For this review, take the finished solid that the model builds, in its own axes (mm). A direction names the side the tool comes from. Coordinates: 2 decimals unless noted, no trailing zeros. Write each loop counter-clockwise with the first axis right and the second up, starting at its lowest first coordinate (ties: lowest second). Pieces come first, ordered by that corner, then holes.
```python
from build123d import *

# Parameters (mm, degrees)
SKETCH2_R               = 5
BOSS_EXTRUDE1_DEPTH     = 8
SKETCH4_R               = 4.55
CUT_EXTRUDE1_DEPTH      = 7.1
CUT_EXTRUDE2_DEPTH      = 11.677078252
CUT_EXTRUDE2_DEPTH_BACK = 11.677078252
SKETCH11_R              = 1.6


with BuildPart() as part:
    # Sketch2 → Boss-Extrude1 (new body)
    with BuildSketch(Plane(origin=(0, 0, 0), x_dir=(1, 0, 0), z_dir=(0, 1, 0))):
        with Locations(Location((0, 0, 0), (0, 0, 270))):
            Circle(SKETCH2_R)
    extrude(amount=BOSS_EXTRUDE1_DEPTH)

    # Sketch4 → Cut-Extrude1 (cut)
    with BuildSketch(Plane(origin=(0, 0, 0), x_dir=(1, 0, 0), z_dir=(0, 1, 0))):
        with Locations(Location((0, 0, 0), (0, 0, 270))):
            Circle(SKETCH4_R)
    extrude(amount=CUT_EXTRUDE1_DEPTH, mode=Mode.SUBTRACT)

    # Sketch11 → Cut-Extrude2 (cut, two sides: drawn at the far end of the back side and taken through both)
    with BuildSketch(Plane.XY.offset(-CUT_EXTRUDE2_DEPTH_BACK)):
        with Locations((0, 2.1)):
            Circle(SKETCH11_R)
    extrude(amount=CUT_EXTRUDE2_DEPTH + CUT_EXTRUDE2_DEPTH_BACK, mode=Mode.SUBTRACT)


solid = part.part
```
Q1. Add section B-B (y = 1.5). State the section outline as (x, z) points.
Ans:
outline: (-1.48, -4.77) - (-1.48, -4.3) arc R4.55 cw to (-1.48, 4.3) - (-1.48, 4.77) arc R5 ccw to start; (1.48, -4.77) arc R5 ccw to (1.48, 4.77) - (1.48, 4.3) arc R4.55 cw to (1.48, -4.3) - close
Q2. Clearance check with flat-ended pins moving along their axes: pin 1 Ø2.5 at (x, z) = (1.5, -1.5) entering from -Y; pin 2 Ø1 at (y, z) = (1.5, 2) entering from +X; pin 3 Ø3 at (x, y) = (0, 2.1) entering from -Z. State where each tip first meets the part, or that it passes through.
Ans:
pin 1: stops at y = 7.1
pin 2: stops at x = 4.77
pin 3: passes through
Q3. Tool access review of faces 4 (the cylindrical face through (-1.27, 1.13, 4.62)), 5 (the cylindrical face through (-1.743, 3.5, 4.203)): name each direction out of +Z, -Z, +X, -X, +Y, -Y from which nothing blocks a thin tool from reaching the whole face with its end or side.
Ans:
face 4: +Z, -Z
face 5: -Y
Q4. Add section D-D (y = 4.25). State the section outline as (x, z) points, then the cut area to 3 significant figures.
Ans:
outline: circle Ø10 at (0, 0); hole circle Ø9.1 at (0, 0)
area: 13.5 mm2
Q5. For probe 1 along Z at (x, y) = (0, 5); probe 2 along Y at (x, z) = (0, -4.5), list the stretches that pass through material, from the lowest coordinate up.
Ans:
probe 1: z = -5 to -4.55, 4.55 to 5
probe 2: y = 7.1 to 8
Q6. Add section A-A (x = 0). State the section outline as (y, z) points, then the cut area to 3 significant figures.
Ans:
outline: (0, -5) - (0.5, -5) - (0.5, -4.55) - (0, -4.55) - close; (0, 4.55) - (0.5, 4.55) - (0.5, 5) - (0, 5) - close; (3.7, -5) - (8, -5) - (8, 5) - (3.7, 5) - (3.7, 4.55) - (7.1, 4.55) - (7.1, -4.55) - (3.7, -4.55) - close
area: 12.5 mm2
Q7. Add section C-C (z = 0). State the section outline as (x, y) points.
Ans:
outline: (-5, 0) - (-4.55, 0) - (-4.55, 7.1) - (4.55, 7.1) - (4.55, 0) - (5, 0) - (5, 8) - (-5, 8) - close
Q8. Draft analysis for pull direction X (two halves, no side actions). For faces 1 (the flat face through (0, 8, 0)), 2 (the cylindrical face through (-1.915, 3.944, 4.619)), 3 (the cylindrical face through (0.86, 3.45, -4.63)), state which applies: +X half, -X half, draft (parallel to the pull), parting line (faces both ways), or undercut.
Ans:
face 1: draft
face 2: parting line
face 3: undercut
